Verification items for the finished model (mm, model axes). Face numbers are marked on the shaded views. A direction names the side the tool comes from. Give positions to 0.01 mm unless a question says otherwise; leave off trailing zeros. Order: outer loops, then holes, each group sorted by start corner. A loop starts at its lowest first (then second) coordinate and runs counter-clockwise, first axis right, second up.
(1) Access from +Z, -Z, +X, -X, +Y, -Y to the whole of each face (thin tool, end or side, straight path). Record for the marked faces 5, 6 and 7.
(2) Sectioned sample at A-A on x = 0. Record the cut outline in (y, z).
(3) Gauge pin test, flat ends, axial feed: pin 1 (2 mm diameter, centred on x = -1.5, y = 15, fed in from -Z); pin 2 (0.6 mm diameter, centred on y = 16, z = 0, fed in from +X); pin 3 (0.6 mm diameter, centred on y = 5, z = 0.5, fed in from -X). Record the tip position at first contact, or that the pin passes through.
(4) Sectioned sample at C-C on y = 9. Record the cut outline in (x, z), plus the area to 3 significant figures.
(5) Scan lines: L1, parallel to Z at x = 0, y = 1.15; L2, parallel to Y at x = 3.5, z = 1; L3, parallel to X at y = 7.5, z = 0.25. Record each from-to range of solid material in increasing order.
(6) Sectioned sample at D-D on z = 4.5. Record the cut outline in (x, y), plus the area to 3 significant figures.
(7) Mould release check, pull along X, two halves, no side actions. Record for the marked faces 1, 2, 3 and 4: pulls with the +X half, pulls with the -X half, needs draft (parallel to the pull), parting line crosses it, or undercut.
(8) Sectioned sample at B-B on z = -7.5. Record the cut outline in (x, y), plus the area to 3 significant figures.
```python
from build123d import *

# Parameters (mm, degrees)
SKETCH1_R           = 10.75
BOSS_EXTRUDE1_DEPTH = 2.6
SKETCH2_R           = 9
BOSS_EXTRUDE2_DEPTH = 10.9
SKETCH3_W           = 6
SKETCH3_H           = 1.2
BOSS_EXTRUDE3_DEPTH = 5
SKETCH4_R           = 9
CUT_EXTRUDE2_DEPTH  = 2
CUT_EXTRUDE3_DEPTH  = 5


with BuildPart() as part:
    # Sketch1 → Boss-Extrude1 (new body)
    with BuildSketch(Plane(origin=(0, 0, 0), x_dir=(1, 0, 0), z_dir=(0, 1, 0))):
        Circle(SKETCH1_R)
    extrude(amount=BOSS_EXTRUDE1_DEPTH)

    # Sketch2 → Boss-Extrude2 (add)
    with BuildSketch(Plane(origin=(0, 2.6, 0), x_dir=(1, 0, 0), z_dir=(0, 1, 0))):
        Circle(SKETCH2_R)
    extrude(amount=BOSS_EXTRUDE2_DEPTH)

    # Sketch3 → Boss-Extrude3 (add)
    with BuildSketch(Plane(origin=(0, 13.5, 0), x_dir=(1, 0, 0), z_dir=(0, 1, 0))):
        Rectangle(SKETCH3_W, SKETCH3_H)
    extrude(amount=BOSS_EXTRUDE3_DEPTH)

    # Sketch4 → Cut-Extrude2 (cut)
    with BuildSketch(Plane.XZ):
        Circle(SKETCH4_R)
    extrude(amount=-CUT_EXTRUDE2_DEPTH, mode=Mode.SUBTRACT)

    # Sketch5 → Cut-Extrude3 (cut)
    with BuildSketch(Plane.XZ.offset(-2)):
        Polygon((-3, 0.9), (-3, -0.2), (-2.3, -0.9), (2.3, -0.9), (3, -0.2), (3, 0.9), align=None)
    extrude(amount=-CUT_EXTRUDE3_DEPTH, mode=Mode.SUBTRACT)


solid = part.part
```
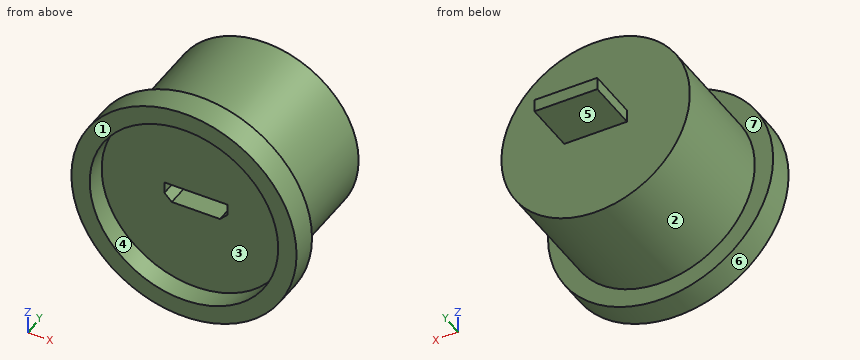
Ans:
1. face 5: -Z, +X, -X, +Y
1. face 6: +Y, -Y
1. face 7: +Y
2. outline: (0, -10.75) - (2.6, -10.75) - (2.6, -9) - (13.5, -9) - (13.5, -0.6) - (18.5, -0.6) - (18.5, 0.6) - (13.5, 0.6) - (13.5, 9) - (2.6, 9) - (2.6, 10.75) - (0, 10.75) - (0, 9) - (2, 9) - (2, 0.9) - (7, 0.9) - (7, -0.9) - (2, -0.9) - (2, -9) - (0, -9) - close
3. pin 1: stops at z = -0.6
3. pin 2: stops at x = 3
3. pin 3: stops at x = -9
4. outline: circle Ø18 at (0, 0)
4. area: 254 mm2
5. L1: z = -10.75 to -9, 9 to 10.75
5. L2: y = 2 to 13.5
5. L3: x = -9 to 9
6. outline: (-9.76, 0) - (-7.79, 0) - (-7.79, 2) - (7.79, 2) - (7.79, 0) - (9.76, 0) - (9.76, 2.6) - (7.79, 2.6) - (7.79, 13.5) - (-7.79, 13.5) - (-7.79, 2.6) - (-9.76, 2.6) - close
6. area: 190 mm2
7. face 1: needs draft
7. face 2: parting line crosses it
7. face 3: undercut
7. face 4: undercut
8. outline: (-7.7, 0) - (-4.97, 0) - (-4.97, 2) - (4.97, 2) - (4.97, 0) - (7.7, 0) - (7.7, 2.6) - (4.97, 2.6) - (4.97, 13.5) - (-4.97, 13.5) - (-4.97, 2.6) - (-7.7, 2.6) - close
8. area: 129 mm2
